from build123d import *

# Parameters (mm, degrees)
F1_DEPTH = 6.35


with BuildPart() as f1:
    # F0 (on Top) → F1 (new body)
    with BuildSketch(Plane.XY):
        with BuildLine():
            ThreePointArc((0, 1.6002), (0.468688, 0.468688), (1.6002, 0))
            Line((1.6002, 0), (42.8498, 0))
            ThreePointArc((42.8498, 0), (43.981312, 0.468688), (44.45, 1.6002))
            Line((44.45, 1.6002), (44.45, 17.4498))
            ThreePointArc((44.45, 17.4498), (44.918688, 18.581312), (46.0502, 19.05))
            Line((46.0502, 19.05), (47.9298, 19.05))
            ThreePointArc((47.9298, 19.05), (49.061312, 19.518688), (49.53, 20.6502))
            Line((49.53, 20.6502), (49.53, 42.8498))
            ThreePointArc((49.53, 42.8498), (49.061312, 43.981312), (47.9298, 44.45))
            Line((47.9298, 44.45), (46.0502, 44.45))
            ThreePointArc((46.0502, 44.45), (44.918688, 44.918688), (44.45, 46.0502))
            Line((44.45, 46.0502), (44.45, 172.9994))
            ThreePointArc((44.45, 172.9994), (44.918688, 174.130912), (46.0502, 174.5996))
            Line((46.0502, 174.5996), (47.9298, 174.5996))
            ThreePointArc((47.9298, 174.5996), (49.061312, 175.068288), (49.53, 176.1998))
            Line((49.53, 176.1998), (49.53, 198.3994))
            ThreePointArc((49.53, 198.3994), (49.061312, 199.530912), (47.9298, 199.9996))
            Line((47.9298, 199.9996), (46.0502, 199.9996))
            ThreePointArc((46.0502, 199.9996), (44.918688, 200.468288), (44.45, 201.5998))
            Line((44.45, 201.5998), (44.45, 217.4494))
            ThreePointArc((44.45, 217.4494), (43.981312, 218.580912), (42.8498, 219.0496))
            Line((42.8498, 219.0496), (1.6002, 219.0496))
            ThreePointArc((1.6002, 219.0496), (0.468688, 218.580912), (0, 217.4494))
            Line((0, 217.4494), (0, 201.5998))
            ThreePointArc((0, 201.5998), (-0.468688, 200.468288), (-1.6002, 199.9996))
            Line((-1.6002, 199.9996), (-3.4798, 199.9996))
            ThreePointArc((-3.4798, 199.9996), (-4.611312, 199.530912), (-5.08, 198.3994))
            Line((-5.08, 198.3994), (-5.08, 176.1998))
            ThreePointArc((-5.08, 176.1998), (-4.611312, 175.068288), (-3.4798, 174.5996))
            Line((-3.4798, 174.5996), (-1.6002, 174.5996))
            ThreePointArc((-1.6002, 174.5996), (-0.468688, 174.130912), (0, 172.9994))
            Line((0, 172.9994), (0, 46.0502))
            ThreePointArc((0, 46.0502), (-0.468688, 44.918688), (-1.6002, 44.45))
            Line((-1.6002, 44.45), (-3.4798, 44.45))
            ThreePointArc((-3.4798, 44.45), (-4.611312, 43.981312), (-5.08, 42.8498))
            Line((-5.08, 42.8498), (-5.08, 20.6502))
            ThreePointArc((-5.08, 20.6502), (-4.611312, 19.518688), (-3.4798, 19.05))
            Line((-3.4798, 19.05), (-1.6002, 19.05))
            ThreePointArc((-1.6002, 19.05), (-0.468688, 18.581312), (0, 17.4498))
            Line((0, 17.4498), (0, 1.6002))
        make_face()
        with BuildLine():
            ThreePointArc((9.525, 26.67), (5.9563, 30.2387), (9.525, 33.8074))
            Line((9.525, 33.8074), (34.925, 33.8074))
            ThreePointArc((34.925, 33.8074), (37.448452, 32.762152), (38.4937, 30.2387))
            ThreePointArc((38.4937, 30.2387), (37.448452, 27.715248), (34.925, 26.67))
            Line((34.925, 26.67), (9.525, 26.67))
        make_face(mode=Mode.SUBTRACT)
        with BuildLine():
            ThreePointArc((9.525, 161.544), (5.9563, 165.1127), (9.525, 168.6814))
            Line((9.525, 168.6814), (34.925, 168.6814))
            ThreePointArc((34.925, 168.6814), (37.448452, 167.636152), (38.4937, 165.1127))
            ThreePointArc((38.4937, 165.1127), (37.448452, 162.589248), (34.925, 161.544))
            Line((34.925, 161.544), (9.525, 161.544))
        make_face(mode=Mode.SUBTRACT)
    extrude(amount=F1_DEPTH)


solid = f1.part
The model under review builds one solid part; all positions refer to its coordinate system, in mm. A direction names the side the tool comes from. Round coordinates to 2 decimals unless told otherwise and drop trailing zeros. Write each loop counter-clockwise with the first axis right and the second up, starting at its lowest first coordinate (ties: lowest second). Pieces come first, ordered by that corner, then holes. Notation, with made-up numbers: (18, 61) -> (76, 61) arc R14 cw to (76, 70) -> close; hole circle Ø9 at (-35.5, 87.25). An arc over 180 degrees is marked (long way). Answer as a JSON object with one key per item and string values.
1. Clearance check with flat-ended pins moving along their axes: pin 1 (1.5 mm diameter, centred on x = 47, z = 4.5, fed in from -Y); pin 2 (0.9 mm diameter, centred on x = -2.5, z = 1.5, fed in from -Y); pin 3 (1.9 mm diameter, centred on y = 118, z = 3.5, fed in from +X). State where each tip first meets the part, or that it passes through.
Results found:
{"pin 1": "stops at y = 19.05", "pin 2": "stops at y = 19.05", "pin 3": "stops at x = 44.45"}
2. To check wall thickness, follow line 1 along Y through (x, z) = (9, 5.25); line 2 along Y through (x, z) = (21.5, 4); line 3 along Y through (x, z) = (-1.5, 0.5). State the ranges of each line that lie inside material, in increasing order.
Results found:
{"line 1": "y = 0 to 26.71, 33.77 to 161.58, 168.64 to 219.05", "line 2": "y = 0 to 26.67, 33.81 to 161.54, 168.68 to 219.05", "line 3": "y = 19.05 to 44.45, 174.6 to 200"}
3. We need section A-A on x = 13. State the section outline as (y, z) points, and give its area (3 significant figures).
Results found:
{"outline": "(0, 0) -> (26.67, 0) -> (26.67, 6.35) -> (0, 6.35) -> close; (33.81, 0) -> (161.54, 0) -> (161.54, 6.35) -> (33.81, 6.35) -> close; (168.68, 0) -> (219.05, 0) -> (219.05, 6.35) -> (168.68, 6.35) -> close", "area": "1,300 mm^2"}
4. We need section B-B on z = 2.75. State how many separate pieces and enclosed holes the cut face has, and give its area (3 significant figures).
Results found:
{"separate pieces": "1", "enclosed holes": "2", "area": "9,810 mm^2"}
5. We need section C-C on y = 146. State the section outline as (x, z) points.
Results found:
{"outline": "(0, 0) -> (44.45, 0) -> (44.45, 6.35) -> (0, 6.35) -> close"}
6. Machinability: for faces 1 (the face through (44.45, 109, 3)), 2 (the face through (5.957, 30.16, 3.131)), 3 (the face through (44.45, 9, 3)), 4 (the face through (0, 210, 3)), 5 (the face through (0, 10, 3)), which of the approach directions +Z, -Z, +X, -X, +Y, -Y give a long, thin tool a straight path to every point of the face, cutting with its end or side? Answer none if there is none.
Results found:
{"face 1": "+Z, -Z, +X", "face 2": "+Z, -Z", "face 3": "+Z, -Z, +X, -Y", "face 4": "+Z, -Z, -X, +Y", "face 5": "+Z, -Z, -X, -Y"}
7. The part is to be moulded in two halves that separate along Y. For faces 6 (the face through (22, 111, 0)), 7 (the face through (0, 110, 3)), 8 (the face through (22, 0, 3)), say which applies: pulls with the +Y half, pulls with the -Y half, needs draft (parallel to the pull), parting line crosses it, or undercut.
Results found:
{"face 6": "needs draft", "face 7": "undercut", "face 8": "pulls with the -Y half"}
